from build123d import *

# Parameters (mm, degrees)
F1_DEPTH = 146.39604
F0_R     = 83.392936441
F2_DEPTH = 535.26303
F3_DEPTH = 314.9086
F4_DEPTH = 317.17995
F0_R_2   = 48.5130356929
F0_R_3   = 50
F5_DEPTH = 145.32376


with BuildPart() as f1:
    # F0 (on Front) → F1 (new body)
    with BuildSketch(Plane.XZ):
        with BuildLine():
            Line((28.9590880275, -175.4914518826), (798.1629728788, -175.4914518826))
            add(Edge.make_bspline(
                [(726.2878835215, 0), (749.4564260521, -3.6950431615), (807.986100889, -13.0296689571), (801.8625568935, -114.3051358252), (798.1629728788, -175.4914518826)],
                knots=[0, 0, 0, 0, 0.3958426661, 1, 1, 1, 1], degree=3))
            Line((726.2878835215, 0), (-295.5661843732, 0))
            ThreePointArc((-295.5661843732, 0), (-667.1886575617, 138.684058053), (-297.4846392131, 282.4041657406))
            Line((-297.4846392131, 282.4041657406), (729.4129350169, 282.4041657406))
            add(Edge.make_bspline(
                [(729.4129350169, 282.4041657406), (747.6261257194, 287.3140311043), (795.952797715, 300.3418117303), (789.6132360534, 396.0934109874), (785.6629066882, 455.7584753077)],
                knots=[0, 0, 0, 0, 0.3768765766, 1, 1, 1, 1], degree=3))
            Line((785.6629066882, 455.7584753077), (-454.9619642401, 455.7584753077))
            ThreePointArc((-454.9619642401, 455.7584753077), (-770.5907953617, 138.5632624305), (-451.8369741687, -175.4914518826))
            Line((-451.8369741687, -175.4914518826), (28.9590880275, -175.4914518826))
        make_face()
    extrude(amount=F1_DEPTH)

    # F0 (on Front) → F2 (join)
    with BuildSketch(Plane.XZ):
        with BuildLine():
            ThreePointArc((-297.4846392131, 282.4041657406), (-667.1886575617, 138.684058053), (-295.5661843732, 0))
            ThreePointArc((-295.5661843732, 0), (-273.656680853, 29.8051433358), (-257.2551892643, 62.9618016028))
            ThreePointArc((-257.2551892643, 62.9618016028), (-246.3931852105, 100.8662258675), (-242.7303739653, 140.1257766123))
            ThreePointArc((-242.7303739653, 140.1257766123), (-245.778146476, 175.9640005668), (-254.8339283377, 210.7729078804))
            ThreePointArc((-254.8339283377, 210.7729078804), (-272.6074802891, 248.703352997), (-297.4846392131, 282.4041657406))
        make_face()
        with Locations((-454.9619642401, 140.1257766123)):
            Circle(F0_R, mode=Mode.SUBTRACT)
    extrude(amount=F2_DEPTH)

    # F0 (on Front) → F3 (join)
    with BuildSketch(Plane.XZ):
        with BuildLine():
            Line((798.1629728788, -175.4914518826), (829.4129794979, -175.4914518826))
            add(Edge.make_bspline(
                [(829.4129794979, -175.4914518826), (847.465214072, -176.203771441), (865.5174486461, -176.9160909994), (883.1099902927, -177.1965162426)],
                knots=[0, 0, 0, 0, 0.1205058402, 0.1205058402, 0.1205058402, 0.1205058402], degree=3))
            add(Edge.make_bspline(
                [(804.4128486555, 62.9618016028), (828.5267205054, 56.4951891145), (893.4177428317, 39.0775894842), (887.0936826735, -93.6873293316), (883.1099902927, -177.1965162426)],
                knots=[0, 0, 0, 0, 0.3715086385, 1, 1, 1, 1], degree=3))
            Line((804.4128486555, 62.9618016028), (-257.2551892643, 62.9618016028))
            ThreePointArc((-257.2551892643, 62.9618016028), (-273.656680853, 29.8051433358), (-295.5661843732, 0))
            Line((-295.5661843732, 0), (726.2878835215, 0))
            add(Edge.make_bspline(
                [(726.2878835215, 0), (749.4564260521, -3.6950431615), (807.986100889, -13.0296689571), (801.8625568935, -114.3051358252), (798.1629728788, -175.4914518826)],
                knots=[0, 0, 0, 0, 0.3958426661, 1, 1, 1, 1], degree=3))
        make_face()
    extrude(amount=F3_DEPTH)

    # F0 (on Front) → F4 (join)
    with BuildSketch(Plane.XZ):
        with BuildLine():
            add(Edge.make_bspline(
                [(804.4128476405, 210.7729078804), (828.9197638548, 216.1039467831), (896.2936796349, 230.7451115899), (880.3220514089, 370.0353389293), (870.172874346, 458.57987889)],
                knots=[0, 0, 0, 0, 0.363835826, 1, 1, 1, 1], degree=3))
            add(Edge.make_bspline(
                [(829.4129794979, 455.7584753077), (843.0623410115, 456.7960447436), (856.7117025252, 457.8336141794), (870.172874346, 458.57987889)],
                knots=[0, 0, 0, 0, 0.0723496884, 0.0723496884, 0.0723496884, 0.0723496884], degree=3))
            Line((829.4129794979, 455.7584753077), (785.6629066882, 455.7584753077))
            add(Edge.make_bspline(
                [(729.4129350169, 282.4041657406), (747.6261257194, 287.3140311043), (795.952797715, 300.3418117303), (789.6132360534, 396.0934109874), (785.6629066882, 455.7584753077)],
                knots=[0, 0, 0, 0, 0.3768765766, 1, 1, 1, 1], degree=3))
            Line((729.4129350169, 282.4041657406), (-297.4846392131, 282.4041657406))
            ThreePointArc((-297.4846392131, 282.4041657406), (-272.6074802891, 248.703352997), (-254.8339283377, 210.7729078804))
            Line((-254.8339283377, 210.7729078804), (804.4128476405, 210.7729078804))
        make_face()
    extrude(amount=F4_DEPTH)

    # F0 (on Front) → F5 (join)
    with BuildSketch(Plane.XZ):
        with BuildLine():
            add(Edge.make_bspline(
                [(804.4128486555, 62.9618016028), (828.5267205054, 56.4951891145), (893.4177428317, 39.0775894842), (887.0936826735, -93.6873293316), (883.1099902927, -177.1965162426)],
                knots=[0, 0, 0, 0, 0.3715086385, 1, 1, 1, 1], degree=3))
            add(Edge.make_bspline(
                [(883.1099902927, -177.1965162426), (943.4852931991, -178.1588990152), (1060.3679465943, -169.3878874077), (1068.7319224793, -58.6605543312), (1073.1629464026, 0)],
                knots=[0.1205058402, 0.1205058402, 0.1205058402, 0.1205058402, 0.5340661288, 1, 1, 1, 1], degree=3))
            add(Edge.make_bspline(
                [(870.172874346, 458.57987889), (932.4516179308, 462.0325076192), (1093.8840254449, 454.3206002683), (1081.2427804982, 177.1546292987), (1073.1629464026, 0)],
                knots=[0.0723496884, 0.0723496884, 0.0723496884, 0.0723496884, 0.4070789192, 1, 1, 1, 1], degree=3))
            add(Edge.make_bspline(
                [(804.4128476405, 210.7729078804), (828.9197638548, 216.1039467831), (896.2936796349, 230.7451115899), (880.3220514089, 370.0353389293), (870.172874346, 458.57987889)],
                knots=[0, 0, 0, 0, 0.363835826, 1, 1, 1, 1], degree=3))
            Line((804.4128476405, 210.7729078804), (-254.8339283377, 210.7729078804))
            ThreePointArc((-254.8339283377, 210.7729078804), (-245.778146476, 175.9640005668), (-242.7303739653, 140.1257766123))
            ThreePointArc((-242.7303739653, 140.1257766123), (-246.3931852105, 100.8662258675), (-257.2551892643, 62.9618016028))
            Line((-257.2551892643, 62.9618016028), (804.4128486555, 62.9618016028))
        make_face()
        with Locations((1001.2879099977, -75.4914651207)):
            Circle(F0_R_2, mode=Mode.SUBTRACT)
        with BuildLine():
            ThreePointArc((960.662880212, 166.9520690404), (1044.7099487557, 128.542793686), (960.662880212, 90.1335183316))
            Line((960.662880212, 90.1335183316), (470.0379563312, 93.2585150221))
            Line((470.0379563312, 93.2585150221), (470.0379563312, 166.9520690404))
            Line((470.0379563312, 166.9520690404), (960.662880212, 166.9520690404))
        make_face(mode=Mode.SUBTRACT)
        with Locations((998.1628669739, 327.6335117126)):
            Circle(F0_R_3, mode=Mode.SUBTRACT)
    extrude(amount=F5_DEPTH)


solid = f1.part
Could you check a few things on this model? Use its own coordinates, in mm. A direction names the side the tool comes from. Coordinates: 2 decimals unless noted, no trailing zeros. Order: outer loops, then holes, each group sorted by start corner. A loop starts at its lowest first (then second) coordinate and runs counter-clockwise, first axis right, second up. Notation, with made-up numbers: (-30.75, 61.5) -> (-11.75, 61.5) arc R7 ccw to (-11.75, 73.5) -> close; hole circle Ø5 at (84, -18). An arc over 180 degrees is marked (long way). One line per question, with ' | ' between items.
Q1. I'm going to push flat-ended pins straight in: P1, Ø4, axis at x = 207.5, z = 135, coming from the +Y side; P2, Ø12, axis at x = 220, z = 185.5, coming from the -Y side; P3, Ø3, axis at x = -361.5, z = 343, coming from the -Y side; P4, Ø2, axis at x = -501, y = -425.5, coming from the +Z side. Where does each tip first touch, or does it pass through?
Return value:
P1: y = 0 | P2: y = -145.32 | P3: y = -146.4 | P4: z = 347.52
Q2. On a 3-axis mill with a long thin cutter (end or side, diameter ignored), from which of +Z, -Z, +X, -X, +Y, -Y can I reach the whole of each face in a straight line? I mean faces 1 (the face through (30, -146.396, 285)), 2 (the face through (384, -314.909, 6)), 3 (the face through (180, -85, -175.491)), 4 (the face through (223, -231, 282.404)), 5 (the face through (267, -230, 210.773)). Say none if no direction works.
Return value:
face 1: -Y | face 2: -Z, +X, -Y | face 3: -Z, -X, +Y, -Y | face 4: +Z, -Y | face 5: +X, -Y
Q3. Imagine slicing it at A-A on x = 316. Please give me the cut outline in (y, z), and give its area (3 significant figures).
Return value:
outline: (-317.18, 210.77) -> (-145.32, 210.77) -> (-145.32, 62.96) -> (-314.91, 62.96) -> (-314.91, 0) -> (-146.4, 0) -> (-146.4, -175.49) -> (0, -175.49) -> (0, 455.76) -> (-146.4, 455.76) -> (-146.4, 282.4) -> (-317.18, 282.4) -> close | area: 115,000 mm²
Q4. Imagine slicing it at B-B on x = -390. Please give me the cut outline in (y, z) (3 decimals), and give its area (3 significant figures).
Return value:
outline: (-535.263, -61.919) -> (-146.396, -61.919) -> (-146.396, -175.491) -> (0, -175.491) -> (0, 87.835) -> (-535.263, 87.835) -> close; (-535.263, 192.417) -> (0, 192.417) -> (0, 455.758) -> (-146.396, 455.758) -> (-146.396, 342.171) -> (-535.263, 342.171) -> close | area: 194,000 mm²
Q5. If I drill on L1, parallel to Z at x = -458, y = -112; L2, parallel to Y at x = -3.5, z = -102.5; L3, parallel to Z at x = 907.5, y = -31, over which ranges is the centre line in solid material (lowest first)?
Return value:
L1: -175.49 to 56.79, 223.46 to 455.74 | L2: -146.4 to 0 | L3: -177.26 to 90.47, 166.95 to 459.67
Q6. Imagine slicing it at C-C on y = -123. State how many separate pieces and enclosed holes the cut face has, and give its area (3 significant figures).
Return value:
separate pieces: 1 | enclosed holes: 4 | area: 1,030,000 mm²
